Autodesk Inventor part; units mm, degrees
ref_plane "YZ Plane" through (0, 0, 0) normal (1, 0, 0) x (0, 1, 0)
ref_plane "XZ Plane" through (0, 0, 0) normal (0, 1, 0) x (-1, 0, 0)
ref_plane "XY Plane" through (0, 0, 0) normal (0, 0, 1) x (1, 0, 0)
sketch "Sketch5" plane through (0, 0, 0) normal (0, 0, 1) x (1, 0, 0)
  line L0 (0, 0) -> (300, 0)
  line L1 (300, 0) -> (300, 500)
  line L2 (300, 500) -> (0, 500)
  line L3 (0, 500) -> (0, 0)
  line L4 (20, 480) -> (280, 480)
  line L5 (280, 480) -> (280, 20)
  line L6 (280, 20) -> (20, 20)
  line L7 (20, 20) -> (20, 480)
  line L8 (150, 0) -> (150, 500)
  circle A0 centre (150, 250) radius 36
  circle A1 centre (114, 250) radius 2
  circle A2 centre (168, 218.8231) radius 2
  circle A3 centre (168, 281.1769) radius 2
  line L9 (20, 250) -> (150, 250)
  line L10 (20, 240) -> (150, 240)
  line L11 (20, 260) -> (150, 260)
  line L12 (280, 20) -> (150, 250)
  line L13 (150, 250) -> (280, 480)
  line L14 (271.2944, 15.0794) -> (141.2944, 245.0794)
  line L15 (288.7056, 24.9206) -> (158.7056, 254.9206)
  line L16 (158.7056, 245.0794) -> (288.7056, 475.0794)
  line L17 (141.2944, 254.9206) -> (271.2944, 484.9206)
  point P0 (161.4868, 250)
  point P1 (280, 459.6772)
  point P2 (280, 40.3228)
  point P3 (144.1654, 240)
  point P4 (268.5132, 20)
  point P5 (268.5132, 480)
  point P6 (144.1654, 260)
  dimension "d31" = 72
  dimension "d28" = 300
  dimension "d29" = 500
  dimension "d30" = 20
  dimension "d32" = 4
  dimension "d35" = 360
  dimension "d37" = 10
  dimension "d38" = 10
  dimension "d39" = 10
  dimension "d40" = 10
  dimension "d41" = 10
  dimension "d42" = 10
extrude "Extrusion5" add sketch "Sketch5" along normal blind 20 contours L3 L2 L8 L4 L7 L6 L0 | L8 L6 L5 L4 L2 L1 L0 | L14 A0 A2 L12 L6 | L12 A2 A0 L15 L5 | L14 L8 L12 A2 A0 | L7 L9 A1 A0 L10 | L14 L10 L8 | A0 A1 L9 L8 L10 | L4 L13 A3 A0 L17 | L12 A0 A2 | A2 A0 L12 | A2 L12 A0 | L7 L11 A0 A1 L9 | A1 L9 A0 | A0 L9 A1 | L5 L16 A0 A3 L13 | A0 A3 L13 L8 L17 | L8 L11 L17 | L11 L8 L9 A1 A0 | A0 A2 L12 L13 A3 L16 L15 | L12 A2 A0 | A1 A0 L9 | A0 A1 L9 | L13 A0 A3 | A3 A0 L13 | A0 L13 A3 | L13 A0 A3
hole "Hole1" at (168, 218.8231, 0) at (168, 281.1769, 0) at (114, 250, 0) direction (0, 0, 1) diameter 4.3 depth 20
fillet "Fillet1" radius 10 15 edges at (0, 0, 10) (20, 20, 10) (300, 0, 10) (268.5132, 20, 10) (280, 40.3228, 10) (144.1654, 240, 10) (144.1654, 260, 10) (161.4868, 250, 10) (20, 240, 10) (20, 260, 10) (0, 500, 10) (20, 480, 10) (300, 500, 10) (268.5132, 480, 10) (280, 459.6772, 10)
properties part number "Aufhängung"
Work out the finished part from the listing and answer in its coordinate system (mm). A direction names the side the tool comes from. Coordinates: 2 decimals unless noted, no trailing zeros. Order: outer loops, then holes, each group sorted by start corner. A loop starts at its lowest first (then second) coordinate and runs counter-clockwise, first axis right, second up. Notation, with made-up numbers: (21.5, 26) - (68.5, 26) arc R16 cw to (68.5, 37) - close; hole circle Ø2 at (19, 46). An arc over 180 degrees is marked (long way). Answer as a JSON object with one key per item and string values.
1. The mould has two halves that part along Y. Classify faces 3 (the face through (160, 251, 20)), 4 (the face through (272.366, 68.622, 10.14)), 5 (the face through (3.01, 497.15, 10.14)): +Y half, -Y half, draft (parallel to the pull), parting line (faces both ways), or undercut.
Output values:
{"face 3": "draft", "face 4": "undercut", "face 5": "+Y half"}
2. Consider line 1 (X direction, y = 250, z = 7); line 2 (Y direction, x = 89, z = 3.25); line 3 (X direction, y = 449.5, z = 18.5). Determine where each line is inside the solid, lowest interval first.
Output values:
{"line 1": "x = 0 to 111.85, 116.15 to 162.97, 280 to 300", "line 2": "y = 0 to 20, 240 to 260, 480 to 500", "line 3": "x = 0 to 20, 251.27 to 300"}
3. Find section B-B on z = 9.5. Count the separate pieces of the cut face and the enclosed holes in it, plus the area to 3 significant figures.
Output values:
{"separate pieces": "1", "enclosed holes": "6", "area": "43,800 mm²"}
4. Each of these flat-tipped pins is pushed along its axis until it touches: P1, Ø3.5, axis at x = 168, y = 281.18, coming from the -Z side; P2, Ø3, axis at x = 69, z = 8.5, coming from the -Y side. Where does it stop, or does it pass through?
Output values:
{"P1": "passes through", "P2": "stops at y = 0"}
5. Find section A-A on x = 54.5. Determine the outline of the cut face in (y, z), plus the area to 3 significant figures.
Output values:
{"outline": "(0, 0) - (20, 0) - (20, 20) - (0, 20) - close; (240, 0) - (260, 0) - (260, 20) - (240, 20) - close; (480, 0) - (500, 0) - (500, 20) - (480, 20) - close", "area": "1,200 mm²"}
6. A tool of negligible diameter and unlimited length cuts with its end or side. For faces 1 (the face through (2.85, 3.01, 10.14)), 2 (the face through (83, 260, 10)), from which of +Z, -Z, +X, -X, +Y, -Y can it reach the whole face along a straight path? Write none if from no direction.
Output values:
{"face 1": "+Z, -Z, -X, -Y", "face 2": "+Z, -Z"}
7. Find section C-C on x = 273.5. Determine the outline of the cut face in (y, z), plus the area to 3 significant figures.
Output values:
{"outline": "(0, 0) - (68.97, 0) - (68.97, 20) - (0, 20) - close; (431.03, 0) - (500, 0) - (500, 20) - (431.03, 20) - close", "area": "2,760 mm²"}
8. Find section D-D on y = 60. Determine the outline of the cut face in (x, z).
Output values:
{"outline": "(0, 0) - (20, 0) - (20, 20) - (0, 20) - close; (245.9, 0) - (300, 0) - (300, 20) - (245.9, 20) - close"}
